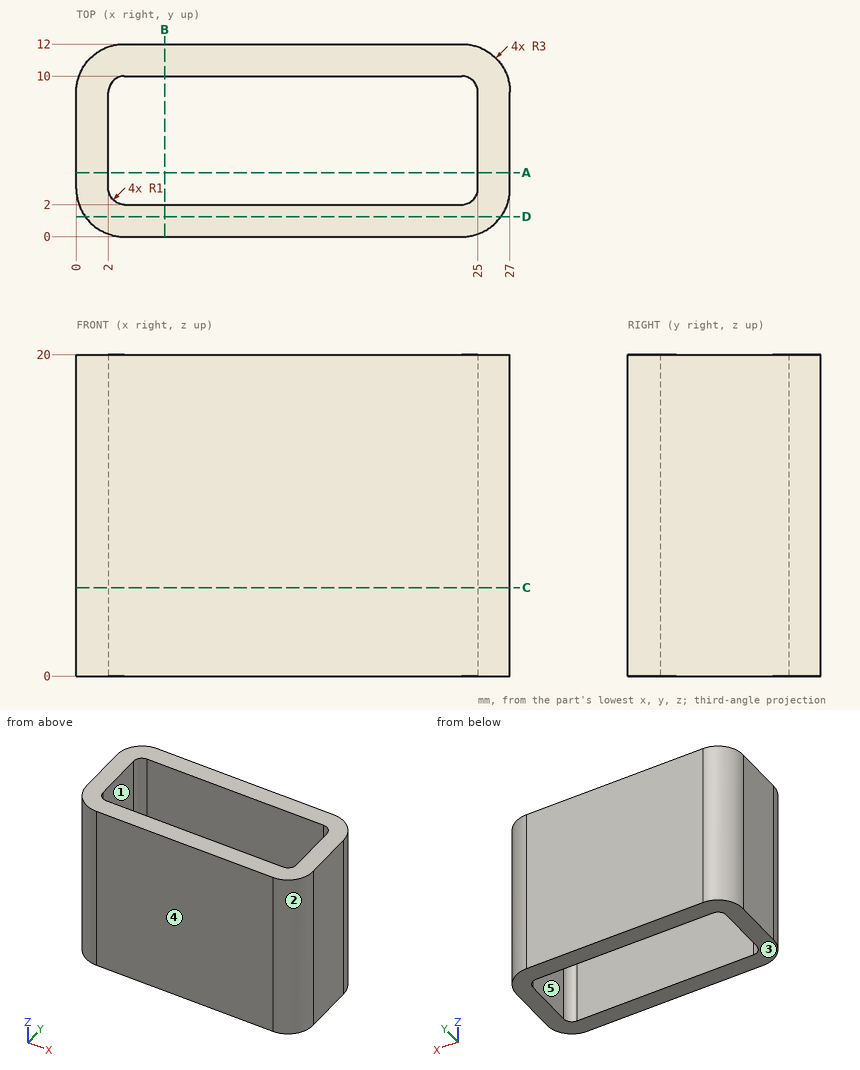
Design review of the part shown in the three views and the two pictorial views. Dimensions are in mm from the part's minimum x, y and z. A direction names the side the tool comes from. Coordinates: 2 decimals unless noted, no trailing zeros. Write each loop counter-clockwise with the first axis right and the second up, starting at its lowest first coordinate (ties: lowest second). Pieces come first, ordered by that corner, then holes.
1) To check wall thickness, follow probe 1 along X at (y, z) = (7, 10.25); probe 2 along Y at (x, z) = (8, 16.5); probe 3 along X at (y, z) = (1.75, 16.75). State the ranges of each line that lie inside material, in increasing order.
2) Machinability: for the marked faces 4 and 5, which of the approach directions +Z, -Z, +X, -X, +Y, -Y give a long, thin tool a straight path to every point of the face, cutting with its end or side? Answer none if there is none.
3) We need section B-B on x = 5.5. State the section outline as (y, z) points, then the cut area to 3 significant figures.
4) The part is to be moulded in two halves that separate along X. For the marked faces 1, 2 and 3, say which applies: pulls with the +X half, pulls with the -X half, needs draft (parallel to the pull), parting line crosses it, or undercut.
5) We need section D-D on y = 1.25. State the section outline as (x, z) points, then the cut area to 3 significant figures.
6) We need section C-C on z = 5.5. State the section outline as (x, y) points, then the cut area to 3 significant figures.
7) We need section A-A on y = 4. State the section outline as (x, z) points.
Answer list:
1. probe 1: x = 0 to 2, 25 to 27
1. probe 2: y = 0 to 2, 10 to 12
1. probe 3: x = 0.27 to 26.73
2. face 4: +Z, -Z, +X, -X, -Y
2. face 5: +Z, -Z
3. outline: (0, 0) - (2, 0) - (2, 20) - (0, 20) - close; (10, 0) - (12, 0) - (12, 20) - (10, 20) - close
3. area: 80.0 mm2
4. face 1: undercut
4. face 2: pulls with the +X half
4. face 3: needs draft
5. outline: (0.56, 0) - (26.44, 0) - (26.44, 20) - (0.56, 20) - close
5. area: 517 mm2
6. outline: (0, 3) arc R3 ccw to (3, 0) - (24, 0) arc R3 ccw to (27, 3) - (27, 9) arc R3 ccw to (24, 12) - (3, 12) arc R3 ccw to (0, 9) - close; hole (2, 3) arc R1 ccw to (3, 2) - (24, 2) arc R1 ccw to (25, 3) - (25, 9) arc R1 ccw to (24, 10) - (3, 10) arc R1 ccw to (2, 9) - close
6. area: 133 mm2
7. outline: (0, 0) - (2, 0) - (2, 20) - (0, 20) - close; (25, 0) - (27, 0) - (27, 20) - (25, 20) - close
